Answer from the drawing. Dimensions are ordinates in mm from the lowest x, y and z of the part. Round coordinates to 2 decimals unless told otherwise and drop trailing zeros. Order: outer loops, then holes, each group sorted by start corner. A loop starts at its lowest first (then second) coordinate and runs counter-clockwise, first axis right, second up.
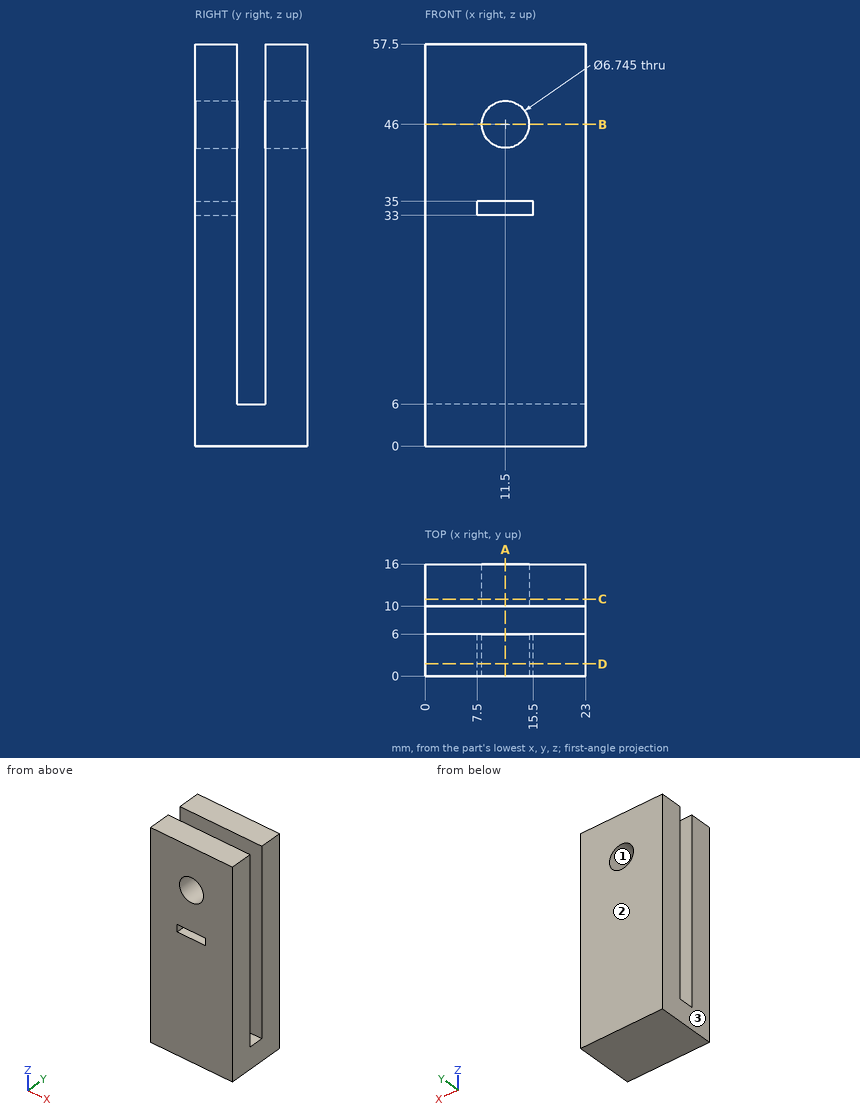
Q1. A cutting plane is placed at B-B, the plane z = 46. Give the vertices of the cut face in (x, y).
Outcome:
outline: (0, 0) - (8.13, 0) - (8.13, 6) - (0, 6) - close; (0, 10) - (8.13, 10) - (8.13, 16) - (0, 16) - close; (14.87, 0) - (23, 0) - (23, 6) - (14.87, 6) - close; (14.87, 10) - (23, 10) - (23, 16) - (14.87, 16) - close
Q2. A cutting plane is placed at D-D, the plane y = 1.75. Give the vertices of the cut face in (x, z) (1 decimal), plus the area to 3 significant figures.
Outcome:
outline: (0, 0) - (23, 0) - (23, 57.5) - (0, 57.5) - close; hole (7.5, 33) - (15.5, 33) - (15.5, 35) - (7.5, 35) - close; hole circle Ø6.7 at (11.5, 46)
area: 1,270 mm2
Q3. A flat-ended cylindrical pin translates along its axis: pin 1 (6 mm diameter, centred on x = 18.5, y = 7, fed in from -Z). Find the tip coordinate at first contact, or state that the pin passes through.
Outcome:
pin 1: stops at z = 0
Q4. A cutting plane is placed at C-C, the plane y = 11. Give the vertices of the cut face in (x, z) (1 decimal).
Outcome:
outline: (0, 0) - (23, 0) - (23, 57.5) - (0, 57.5) - close; hole circle Ø6.7 at (11.5, 46)
Q5. A cutting plane is placed at A-A, the plane x = 11.5. Give the vertices of the cut face in (y, z), plus the area to 3 significant figures.
Outcome:
outline: (0, 0) - (16, 0) - (16, 42.63) - (10, 42.63) - (10, 6) - (6, 6) - (6, 33) - (0, 33) - close; (0, 35) - (6, 35) - (6, 42.63) - (0, 42.63) - close; (0, 49.37) - (6, 49.37) - (6, 57.5) - (0, 57.5) - close; (10, 49.37) - (16, 49.37) - (16, 57.5) - (10, 57.5) - close
area: 621 mm2
Q6. Straight lines are drawn through the part: probe 1 along Z at (x, y) = (11.5, 1.55); probe 2 along Y at (x, z) = (4.5, 27); probe 3 along Z at (x, y) = (11.5, 12.5). For each, find the intervals that lie inside material, in ascending order.
Outcome:
probe 1: z = 0 to 33, 35 to 42.63, 49.37 to 57.5
probe 2: y = 0 to 6, 10 to 16
probe 3: z = 0 to 42.63, 49.37 to 57.5
Q7. For a pull along X with two mould halves and no side action, classify the marked faces 1, 2 and 3 as released by +X, released by -X, zero draft, split by the parting line, or undercut.
Outcome:
face 1: undercut
face 2: zero draft
face 3: released by -X
